Check sheet for the modelled part. Datum: model origin and axes. Units: mm. Give positions to 0.01 mm unless a question says otherwise; leave off trailing zeros. Loops run counter-clockwise (first coordinate to the right, second up) from the corner with the lowest first, then second, coordinate; pieces in that order, holes last. Notation, with made-up numbers: (87.25, 27.25) -> (129.25, 27.25) arc R21 cw to (129.25, 44.25) -> close; hole circle Ø8 at (8.5, 36). An arc over 180 degrees is marked (long way). Write each question's results on one line, items separated by ' | '. Start each with the question number.
Item 1: Cross-section at A-A on x = 114.5. Enter the section's corners in (y, z), then the cut area to 3 significant figures.
Item 2: Cross-section at B-B on z = 1.3. State how many separate pieces and enclosed holes the cut face has, then the cut area to 3 significant figures.
Item 3: Scan lines: line 1 along Y through (x, z) = (118, 1.25); line 2 along Y through (x, z) = (98.5, 1.15); line 3 along Y through (x, z) = (77, 1). Record each from-to range of solid material in increasing order.
Item 4: Gauge pin test, flat end, axial feed: pin 1 Ø1.9 at (x, y) = (62.75, -166) entering from +Z. Record the tip position at first contact, or that the pin passes through.
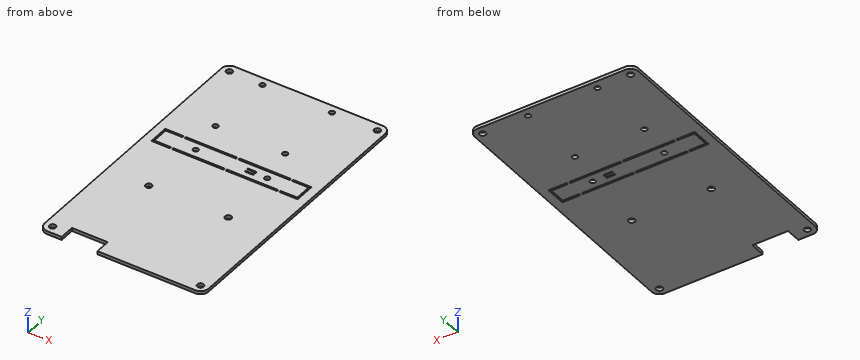
from build123d import *

# Parameters (mm, degrees)
MODEL_R             = 1.3
MODEL_R_2           = 1.35
MODEL_R_3           = 1.6
MODEL_W             = 25.800871102
MODEL_H             = 0.899853509
MODEL_W_2           = 25.800870102
MODEL_H_2           = 0.900030515
BOSS_EXTRUDE1_DEPTH = 1.6


with BuildPart() as part:
    # Model → Boss-Extrude1 (new body)
    with BuildSketch(Plane.XY):
        with BuildLine():
            Line((70.002361624, -162.304686543), (88.002880425, -162.304686543))
            Line((88.002880425, -162.304686543), (88.002880425, -169.986796467))
            Line((88.002880425, -169.986796467), (137.258712697, -169.986796467))
            add(Edge.make_bspline(
                [(137.258712697, -169.986796467), (138.316181375, -169.986784466), (139.330341633, -169.566711691), (140.078087155, -168.81897017)],
                knots=[0, 0, 0, 0, 1, 1, 1, 1], degree=3))
            add(Edge.make_bspline(
                [(140.078087155, -168.81897017), (140.825832676, -168.071228648), (141.245910452, -167.057070391), (141.246087457, -165.999601713)],
                knots=[0, 0, 0, 0, 1, 1, 1, 1], degree=3))
            Line((141.246087457, -165.999601713), (141.246264463, -33.963752791))
            add(Edge.make_bspline(
                [(141.246264463, -33.963752791), (141.246219462, -32.906240112), (140.826140686, -31.892031852), (140.078372164, -31.14425033)],
                knots=[0, 0, 0, 0, 1, 1, 1, 1], degree=3))
            add(Edge.make_bspline(
                [(140.078372164, -31.14425033), (139.330603642, -30.396469808), (138.316402383, -29.976373031), (137.258889703, -29.976735043)],
                knots=[0, 0, 0, 0, 1, 1, 1, 1], degree=3))
            Line((137.258889703, -29.976735043), (62.730494654, -29.976735043))
            add(Edge.make_bspline(
                [(62.730494654, -29.976735043), (61.673022976, -29.976726043), (60.658862718, -30.396804818), (59.911117197, -31.14455134)],
                knots=[0, 0, 0, 0, 1, 1, 1, 1], degree=3))
            add(Edge.make_bspline(
                [(59.911117197, -31.14455134), (59.163396148, -31.892320333), (58.743351208, -32.906494777), (58.743388403, -33.963966454)],
                knots=[0, 0, 0, 0, 1, 1, 1, 1], degree=3))
            Line((58.743388403, -33.963966454), (58.743211397, -165.999601713))
            add(Edge.make_bspline(
                [(58.743211397, -165.999601713), (58.743209397, -168.201763929), (60.52841994, -169.986947472), (62.730583157, -169.986616461)],
                knots=[0, 0, 0, 0, 1, 1, 1, 1], degree=3))
            Line((62.730583157, -169.986616461), (70.002361624, -169.986796467))
            Line((70.002361624, -169.986796467), (70.002361624, -162.304686543))
        make_face()
        with Locations((118.003980767, -87.700241)):
            Circle(MODEL_R, mode=Mode.SUBTRACT)
        with Locations((82.00276616, -87.700241)):
            Circle(MODEL_R, mode=Mode.SUBTRACT)
        with Locations((114.503861986, -69.193633103)):
            Circle(MODEL_R_2, mode=Mode.SUBTRACT)
        with Locations((79.502681173, -69.193633103)):
            Circle(MODEL_R_2, mode=Mode.SUBTRACT)
        with Locations((79.502681173, -34.192456291)):
            Circle(MODEL_R_2, mode=Mode.SUBTRACT)
        with Locations((114.503861986, -34.192456291)):
            Circle(MODEL_R_2, mode=Mode.SUBTRACT)
        with Locations((62.752116863, -34.000356992)):
            Circle(MODEL_R_3, mode=Mode.SUBTRACT)
        with Locations((137.254631064, -34.000356992)):
            Circle(MODEL_R_3, mode=Mode.SUBTRACT)
        with Locations((137.254631064, -166.004811883)):
            Circle(MODEL_R_3, mode=Mode.SUBTRACT)
        with Locations((62.752116863, -166.004811883)):
            Circle(MODEL_R_3, mode=Mode.SUBTRACT)
        with Locations((79.970369511, -119.70654813)):
            Circle(MODEL_R_3, mode=Mode.SUBTRACT)
        with Locations((120.007632474, -119.70654813)):
            Circle(MODEL_R_3, mode=Mode.SUBTRACT)
        Polygon((72.414426725, -82.550246114), (63.175439746, -82.550246114), (63.175439746, -92.850417893), (72.414426725, -92.850417893), (72.414426725, -91.950387378), (63.975466981, -91.950387378), (63.975466981, -83.450099623), (72.414426725, -83.450099623), align=None, mode=Mode.SUBTRACT)
        with Locations((86.514902629, -83.000172869)):
            Rectangle(MODEL_W, MODEL_H, mode=Mode.SUBTRACT)
        with Locations((113.515809584, -83.000172869)):
            Rectangle(MODEL_W_2, MODEL_H, mode=Mode.SUBTRACT)
        with Locations((86.514902629, -92.400402636)):
            Rectangle(MODEL_W, MODEL_H_2, mode=Mode.SUBTRACT)
        with Locations((113.515809584, -92.400402636)):
            Rectangle(MODEL_W_2, MODEL_H_2, mode=Mode.SUBTRACT)
        Polygon((127.616285988, -91.950387378), (127.616285988, -92.850417893), (136.80289525, -92.850417893), (136.80289525, -82.550246114), (127.616285988, -82.550246114), (127.616285988, -83.450099623), (136.002869014, -83.450099623), (136.002869014, -91.950387378), align=None, mode=Mode.SUBTRACT)
        Polygon((107.453624783, -86.436359553), (111.85377408, -86.436359553), (111.85377408, -88.964126448), (107.453624783, -88.964126448), (107.453624783, -88.364106771), (111.253753403, -88.364106771), (111.253753403, -87.03638023), (107.453624783, -87.03638023), align=None, mode=Mode.SUBTRACT)
    extrude(amount=BOSS_EXTRUDE1_DEPTH)


solid = part.part
Answer sheet:
1) outline: (-169.99, 0) -> (-92.85, 0) -> (-92.85, 1.6) -> (-169.99, 1.6) -> close; (-91.95, 0) -> (-83.45, 0) -> (-83.45, 1.6) -> (-91.95, 1.6) -> close; (-82.55, 0) -> (-70.54, 0) -> (-70.54, 1.6) -> (-82.55, 1.6) -> close; (-67.84, 0) -> (-35.54, 0) -> (-35.54, 1.6) -> (-67.84, 1.6) -> close; (-32.84, 0) -> (-29.98, 0) -> (-29.98, 1.6) -> (-32.84, 1.6) -> close | area: 212 mm²
2) separate pieces: 1 | enclosed holes: 19 | area: 11,200 mm²
3) line 1: y = -169.99 to -92.85, -91.95 to -89, -86.4 to -83.45, -82.55 to -29.98 | line 2: y = -169.99 to -92.85, -91.95 to -83.45, -82.55 to -29.98 | line 3: y = -162.3 to -92.85, -91.95 to -83.45, -82.55 to -29.98
4) pin 1: passes through
